Can you work these out from the model? Positions are in its coordinate system, mm. A direction names the side the tool comes from. Give positions to 0.01 mm unless a question says otherwise; leave off trailing zeros. Loops run counter-clockwise (first coordinate to the right, second up) from the corner with the lowest first, then second, coordinate; pieces in that order, holes last. Notation, with made-up numbers: M 11.25,-10.5 L 38.25,-10.5 A19 ccw 38.25,11.5 Z; hole C -22.75,80.25 d6. An arc over 180 degrees is marked long. Use CSV: the item, a comma, the result in double quotes.
from build123d import *

# Parameters (mm, degrees)
SKETCH1_W           = 76.2
SKETCH1_H           = 76.2
BOSS_EXTRUDE1_DEPTH = 184.15
SKETCH3_W           = 76.2
SKETCH3_H           = 76.2
SKETCH3_W_2         = 71.628
SKETCH3_H_2         = 71.628
SKETCH3_W_3         = 68.072
SKETCH3_H_3         = 68.072
CUT_EXTRUDE2_DEPTH  = 12.192
SKETCH4_R           = 30.48
CUT_EXTRUDE4_DEPTH  = 165.1


with BuildPart() as part:
    # Sketch1 → Boss-Extrude1 (new body)
    with BuildSketch(Plane.XY):
        with Locations((38.1, 38.1)):
            Rectangle(SKETCH1_W, SKETCH1_H)
    extrude(amount=-BOSS_EXTRUDE1_DEPTH)

    # Sketch3 → Cut-Extrude2 (cut)
    # profile 1 of 2: a face of its own
    with BuildSketch(Plane.XY):
        with Locations((38.1, 38.1)):
            Rectangle(SKETCH3_W, SKETCH3_H)
        with Locations((38.1, 38.1)):
            Rectangle(SKETCH3_W_2, SKETCH3_H_2, mode=Mode.SUBTRACT)
    # profile 2 of 2: a face of its own
    with BuildSketch(Plane.XY):
        with Locations((38.1, 38.1)):
            Rectangle(SKETCH3_W_3, SKETCH3_H_3)
    extrude(amount=-CUT_EXTRUDE2_DEPTH, mode=Mode.SUBTRACT)

    # Sketch4 → Cut-Extrude4 (cut)
    with BuildSketch(Plane.XY.offset(-12.192)):
        with Locations((44.45, 44.45)):
            Circle(SKETCH4_R)
    extrude(amount=-CUT_EXTRUDE4_DEPTH, mode=Mode.SUBTRACT)


solid = part.part
Q1. For faces 1 (the flat face through (2.286, 38, -6)), 2 (the flat face through (4.064, 38, -6)), 3 (the flat face through (73.914, 38, -6)), 4 (the flat face through (38, 73.914, -6)), 5 (the cylindrical face through (72.606, 32.776, -93.586)), which set-ups out of +Z, -Z, +X, -X, +Y, -Y let a thin tool reach every point of the face, with its end or its side?
Model answer:
face 1,"+Z, -X, +Y, -Y"
face 2,"+Z"
face 3,"+Z, +X, +Y, -Y"
face 4,"+Z, +X, -X, +Y"
face 5,"none"
Q2. Please list where these lines run through material, in increasing order: L1, parallel to X at y = 44.45, z = -108; L2, parallel to Z at x = 72.5, y = 33. Write a range as from..to.
Model answer:
L1,"0..13.97, 74.93..76.2"
L2,"-184.15..-177.29, -12.19..0"
Q3. If we mould it in two halves opening along X, with no side actions, what happens to faces 6 (the flat face through (20, 26, -12.192)), 7 (the flat face through (38, 2.286, -6)), 8 (the flat face through (0, 38, -97))? For each: released by +X, released by -X, zero draft, split by the parting line, or undercut.
Model answer:
face 6,"undercut"
face 7,"zero draft"
face 8,"released by -X"
Q4. I want a section at D-D, the plane x = 59. Please give me the cut outline in (y, z), then the cut area to 3 significant figures.
Model answer:
outline,"M 0,-184.15 L 76.2,-184.15 L 76.2,-12.19 L 73.91,-12.19 L 73.91,0 L 72.14,0 L 72.14,-12.19 L 71.23,-12.19 L 71.23,-177.29 L 17.67,-177.29 L 17.67,-12.19 L 4.06,-12.19 L 4.06,0 L 2.29,0 L 2.29,-12.19 L 0,-12.19 Z"
area,"4,300 mm2"
Q5. I want a section at C-C, the plane z = -121. Please give me the cut outline in (x, y), then the cut area to 3 significant figures.
Model answer:
outline,"M 0,0 L 76.2,0 L 76.2,76.2 L 0,76.2 Z; hole C 44.45,44.45 d60.96"
area,"2,890 mm2"
Q6. I'm going to push flat-ended pins straight in: P1, Ø16.5, axis at x = 68, y = 67, coming from the +Z side; P2, Ø6, axis at x = 40.5, z = -6.5, coming from the -Y side; P3, Ø3.5, axis at y = 47, z = -5, coming from the +X side; P4, Ø6, axis at y = 22.5, z = -6.5, coming from the -X side. Where does each tip first touch, or does it pass through?
Model answer:
P1,"z = 0"
P2,"y = 2.29"
P3,"x = 73.91"
P4,"x = 2.29"
Q7. I want a section at A-A, the plane x = 44.45. Please give me the cut outline in (y, z).
Model answer:
outline,"M 0,-184.15 L 76.2,-184.15 L 76.2,-12.19 L 74.93,-12.19 L 74.93,-177.29 L 13.97,-177.29 L 13.97,-12.19 L 4.06,-12.19 L 4.06,0 L 2.29,0 L 2.29,-12.19 L 0,-12.19 Z; M 72.14,-12.19 L 73.91,-12.19 L 73.91,0 L 72.14,0 Z"
